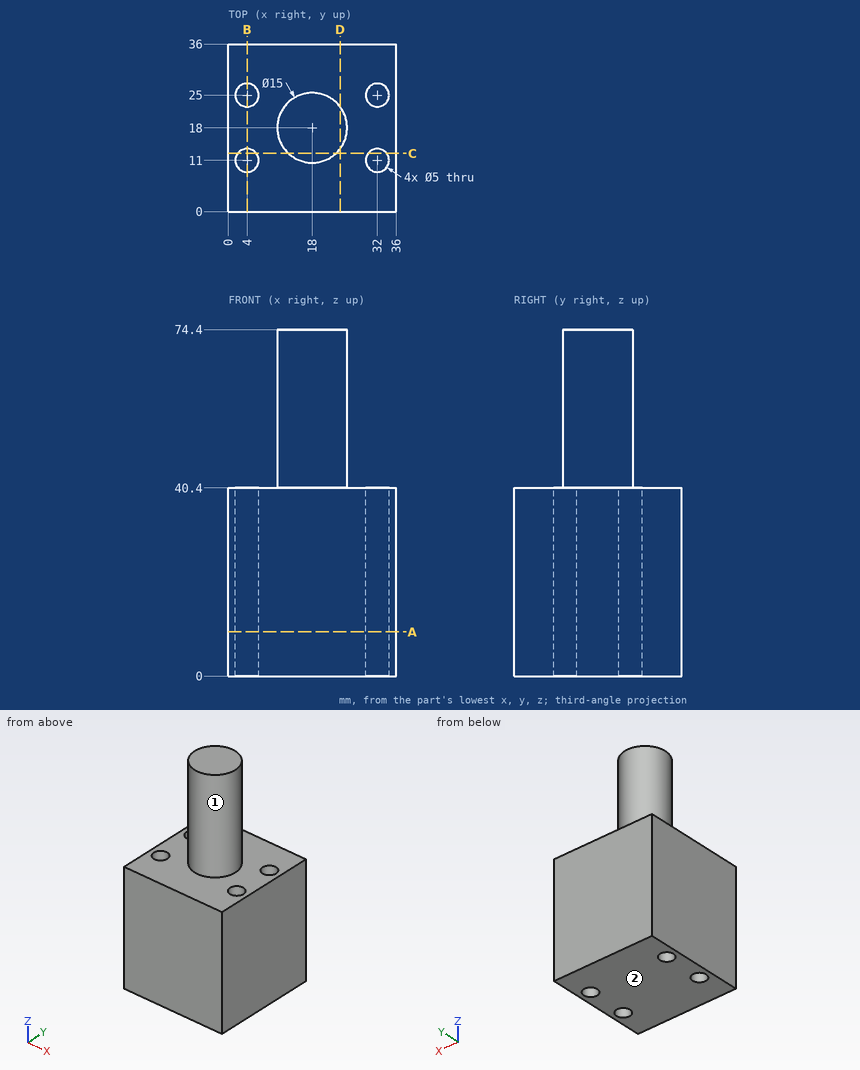
Geometry check sheet. Reference: drawing and pictorial views, mm from the part's lowest x, y, z. A direction names the side the tool comes from. Round coordinates to 2 decimals unless told otherwise and drop trailing zeros. Loops run counter-clockwise (first coordinate to the right, second up) from the corner with the lowest first, then second, coordinate; pieces in that order, holes last. Notation, with made-up numbers: (46.5, 78) -> (52.5, 78) arc R13 cw to (52.5, 100) -> close; hole circle Ø5 at (-37.5, -27). An arc over 180 degrees is marked (long way). Use a Markdown table: item, result.
(1) Sectioned sample at D-D (x = 24). Enter the section's corners in (y, z), then the cut area to 3 significant figures.
Calculated:
| item | result |
|---|---|
| outline | (0, 0) -> (36, 0) -> (36, 40.4) -> (22.5, 40.4) -> (22.5, 74.4) -> (13.5, 74.4) -> (13.5, 40.4) -> (0, 40.4) -> close |
| area | 1,760 mm² |
(2) Sectioned sample at B-B (x = 4). Enter the section's corners in (y, z), then the cut area to 3 significant figures.
Calculated:
| item | result |
|---|---|
| outline | (0, 0) -> (8.5, 0) -> (8.5, 40.4) -> (0, 40.4) -> close; (13.5, 0) -> (22.5, 0) -> (22.5, 40.4) -> (13.5, 40.4) -> close; (27.5, 0) -> (36, 0) -> (36, 40.4) -> (27.5, 40.4) -> close |
| area | 1,050 mm² |
(3) Scan lines: probe 1 along X at (y, z) = (11, 20); probe 2 along Y at (x, z) = (32, 10); probe 3 along X at (y, z) = (23.5, 29.5). Record each from-to range of solid material in increasing order.
Calculated:
| item | result |
|---|---|
| probe 1 | 0 to 1.5, 6.5 to 29.5, 34.5 to 36 |
| probe 2 | 0 to 8.5, 13.5 to 22.5, 27.5 to 36 |
| probe 3 | 0 to 2, 6 to 30, 34 to 36 |
(4) Set-up check for the marked faces 1 and 2: record each of +Z, -Z, +X, -X, +Y, -Y from which the full face is reachable in a straight line by a thin tool's end or side.
Calculated:
| item | result |
|---|---|
| face 1 | +Z |
| face 2 | -Z, +X, -X, +Y, -Y |
(5) Sectioned sample at A-A (z = 9.5). Enter the section's corners in (x, y).
Calculated:
| item | result |
|---|---|
| outline | (0, 0) -> (36, 0) -> (36, 36) -> (0, 36) -> close; hole circle Ø5 at (4, 11); hole circle Ø5 at (4, 25); hole circle Ø5 at (32, 11); hole circle Ø5 at (32, 25) |
(6) Sectioned sample at C-C (y = 12.5). Enter the section's corners in (x, z), then the cut area to 3 significant figures.
Calculated:
| item | result |
|---|---|
| outline | (0, 0) -> (2, 0) -> (2, 40.4) -> (0, 40.4) -> close; (6, 0) -> (30, 0) -> (30, 40.4) -> (23.1, 40.4) -> (23.1, 74.4) -> (12.9, 74.4) -> (12.9, 40.4) -> (6, 40.4) -> close; (34, 0) -> (36, 0) -> (36, 40.4) -> (34, 40.4) -> close |
| area | 1,480 mm² |
(7) Go/stop test with a flat-tipped pin: P1, Ø4, axis at y = 17, z = 50, coming from the -X side. Record where the tip stops, or that it passes through.
Calculated:
| item | result |
|---|---|
| P1 | x = 10.5 |
